```python
from build123d import *

# Parameters (mm, degrees)
BOSS_EXTRUDE1_DEPTH = 1.778
SKETCH3_R           = 1.27
CUT_EXTRUDE1_DEPTH  = 1.778
BOSS_EXTRUDE2_DEPTH = 40.894
SKETCH8_W           = 28.194
SKETCH8_H           = 3.556
CUT_EXTRUDE3_DEPTH  = 3.175
SKETCH10_W          = 28.194
SKETCH10_H          = 1.974840954
CUT_EXTRUDE4_DEPTH  = 31.75


with BuildPart() as part:
    # Sketch1 → Boss-Extrude1 (new body)
    with BuildSketch(Plane.XY):
        with BuildLine():
            Line((-30.353, 12.065), (-30.353, -11.557))
            ThreePointArc((-30.353, -11.557), (-29.311471714, -14.071471714), (-26.797, -15.113))
            Line((-26.797, -15.113), (-4.064, -15.113))
            ThreePointArc((-4.064, -15.113), (-0.254, -18.923), (3.556, -15.113))
            Line((3.556, -15.113), (26.797, -15.113))
            ThreePointArc((26.797, -15.113), (28.989103251, -13.90765993), (29.845, -11.557))
            Line((29.845, -11.557), (29.845, 12.065))
            Line((29.845, 12.065), (28.067, 12.065))
            ThreePointArc((28.067, 12.065), (27.546235857, 13.322235857), (26.289, 13.843))
            Line((26.289, 13.843), (-26.797, 13.843))
            ThreePointArc((-26.797, 13.843), (-28.054235857, 13.322235857), (-28.575, 12.065))
            Line((-28.575, 12.065), (-30.353, 12.065))
        make_face()
    extrude(amount=BOSS_EXTRUDE1_DEPTH)

    # Sketch3 → Cut-Extrude1 (cut)
    with BuildSketch(Plane(origin=(0, 0, 0), x_dir=(-1, 0, 0), z_dir=(0, 0, -1))):
        with Locations((0.254, -16.51)):
            Circle(SKETCH3_R)
    extrude(amount=-CUT_EXTRUDE1_DEPTH, mode=Mode.SUBTRACT)

    # Sketch7 → Boss-Extrude2 (add)
    with BuildSketch(Plane.ZY.offset(20.701)):
        with BuildLine():
            Line((2.032, 14.351), (2.032, 17.399))
            Line((2.032, 17.399), (3.81, 17.399))
            Line((3.81, 17.399), (3.81, 14.351))
            ThreePointArc((3.81, 14.351), (3.140446102, 12.734553898), (1.524, 12.065))
            Line((1.524, 12.065), (1.524, 13.843))
            ThreePointArc((1.524, 13.843), (1.883210245, 13.991789755), (2.032, 14.351))
        make_face()
    extrude(amount=-BOSS_EXTRUDE2_DEPTH)

    # Sketch8 → Cut-Extrude3 (cut, symmetric)
    with BuildSketch(Plane.XY.offset(1.778)):
        with Locations((-0.254, 15.621)):
            Rectangle(SKETCH8_W, SKETCH8_H)
    extrude(amount=CUT_EXTRUDE3_DEPTH, both=True, mode=Mode.SUBTRACT)

    # Sketch10 → Cut-Extrude4 (cut)
    with BuildSketch(Plane.XZ.offset(15.113)):
        with Locations((-0.254, 2.765420477)):
            Rectangle(SKETCH10_W, SKETCH10_H)
    extrude(amount=-CUT_EXTRUDE4_DEPTH, mode=Mode.SUBTRACT)


solid = part.part
```
Input: part model. Units: mm. Frame: model coordinates. A direction names the side the tool comes from. Give positions to 0.01 mm unless a question says otherwise; leave off trailing zeros. Order: outer loops, then holes, each group sorted by start corner. A loop starts at its lowest first (then second) coordinate and runs counter-clockwise, first axis right, second up. Notation, with made-up numbers: (-16.5, 57.25) - (-11.5, 57.25) arc R9 ccw to (-11.5, 66.25) - close; hole circle Ø7 at (-16.75, -27). An arc over 180 degrees is marked (long way). Use a Markdown table: item, result.
(1) Pin query (flat end, axial travel): pin 1 (0.7 mm diameter, centred on y = 13.5, z = 3, fed in from +X); pin 2 (1.4 mm diameter, centred on x = -16.5, z = 1, fed in from -Y); pin 3 (1.5 mm diameter, centred on x = 6, y = -3, fed in from +Z). Return the tip coordinate at first contact, or that it passes through.
Computed values:
| item | result |
|---|---|
| pin 1 | stops at x = 20.19 |
| pin 2 | stops at y = -15.11 |
| pin 3 | stops at z = 1.78 |
(2) Section query A-A (z = 3.2). Output: boundary loops of the cut face in (x, y), then the cut area to 3 significant figures.
Computed values:
| item | result |
|---|---|
| outline | (-20.7, 12.8) - (-14.35, 12.8) - (-14.35, 17.4) - (-20.7, 17.4) - close; (13.84, 12.8) - (20.19, 12.8) - (20.19, 17.4) - (13.84, 17.4) - close |
| area | 58.5 mm2 |
(3) Draft query along X for faces 1 (the flat face through (29.845, 0, 1)), 2 (the flat face through (-30.353, 0, 1)), 3 (the cylindrical face through (-0.09, -15.25, 0.88)). Return one class per face: released by +X, released by -X, zero draft, split by the parting line, or undercut.
Computed values:
| item | result |
|---|---|
| face 1 | released by +X |
| face 2 | released by -X |
| face 3 | undercut |
(4) Section query D-D (y = -16.51). Output: boundary loops of the cut face in (x, z), then the cut area to 3 significant figures.
Computed values:
| item | result |
|---|---|
| outline | (-3.8, 0) - (-1.52, 0) - (-1.52, 1.78) - (-3.8, 1.78) - close; (1.02, 0) - (3.29, 0) - (3.29, 1.78) - (1.02, 1.78) - close |
| area | 8.09 mm2 |
(5) Section query C-C (z = 0.7). Output: boundary loops of the cut face in (x, y) (3 decimals), then the cut area to 3 significant figures.
Computed values:
| item | result |
|---|---|
| outline | (-30.353, -11.557) arc R3.556 ccw to (-26.797, -15.113) - (-4.064, -15.113) arc R3.81 ccw to (3.556, -15.113) - (26.797, -15.113) arc R3.556 ccw to (29.845, -11.557) - (29.845, 12.065) - (28.067, 12.065) arc R1.778 ccw to (26.289, 13.843) - (-26.797, 13.843) arc R1.778 ccw to (-28.575, 12.065) - (-30.353, 12.065) - close; hole circle Ø2.54 at (-0.254, -16.51) |
| area | 1,750 mm2 |
(6) Access query for faces 4 (the flat face through (-29, 12.065, 1)), 5 (the flat face through (-16, -15.113, 1)), 6 (the flat face through (17, 16, 2.032)). Directions: +Z, -Z, +X, -X, +Y, -Y. A direction counts if a zero-diameter tool reaches every point of the face in a straight line with its end or side. Return the directions, or none.
Computed values:
| item | result |
|---|---|
| face 4 | +Z, -Z, -X, +Y |
| face 5 | +Z, -Z, -X, -Y |
| face 6 | -Z, +X, -X, +Y |
(7) Section query B-B (x = 19). Output: boundary loops of the cut face in (y, z), then the cut area to 3 significant figures.
Computed values:
| item | result |
|---|---|
| outline | (-15.11, 0) - (13.84, 0) - (13.84, 1.52) arc R0.51 cw to (14.35, 2.03) - (17.4, 2.03) - (17.4, 3.81) - (14.35, 3.81) arc R2.29 ccw to (12.08, 1.78) - (-15.11, 1.78) - close |
| area | 60.4 mm2 |
(8) Line query: line 1 (X direction, y = 15.5, z = 3.55); line 2 (Z direction, x = -3.5, y = -7); line 3 (Y direction, x = -5.5, z = 0.7). Output: solid intervals per line, ascending. Write a range as from..to.
Computed values:
| item | result |
|---|---|
| line 1 | x = -20.7..-14.35, 13.84..20.19 |
| line 2 | z = 0..1.78 |
| line 3 | y = -15.11..13.84 |
